Geometry check sheet. Reference: the model listing, model coordinates, mm. A direction names the side the tool comes from. Give positions to 0.01 mm unless a question says otherwise; leave off trailing zeros. Order: outer loops, then holes, each group sorted by start corner. A loop starts at its lowest first (then second) coordinate and runs counter-clockwise, first axis right, second up.
Autodesk Inventor part; units mm, degrees
ref_plane "YZ Plane" through (0, 0, 0) normal (1, 0, 0) x (0, 1, 0)
ref_plane "XZ Plane" through (0, 0, 0) normal (0, 1, 0) x (-1, 0, 0)
ref_plane "XY Plane" through (0, 0, 0) normal (0, 0, 1) x (1, 0, 0)
sketch "Sketch1" plane through (0, 0, 0) normal (0, 1, 0) x (-1, 0, 0)
  line L0 (-12, 184.4696) -> (80, 184.4696)
  line L1 (80, 184.4696) -> (80, -38.9934)
  line L2 (80, -38.9934) -> (-12, -38.9934)
  line L3 (-12, -38.9934) -> (-12, 184.4696)
  point P0 (0, 0)
  dimension "d0" = 92
  dimension "d1" = 223.463
extrude "Extrusion1" add sketch "Sketch1" along normal blind 5
sketch "Sketch2" plane through (0, 5, 0) normal (0, 1, 0) x (1, 0, 0)
  line L0 (-80, -184.4696) -> (12, -184.4696)
  line L1 (12, -184.4696) -> (-13, -184.4696)
  line L2 (-13, -184.4696) -> (-13, -154.4696)
  circle A0 centre (-13, -154.4696) radius 4.75
  line L3 (-13, -154.4696) -> (-13, -114.4696)
  line L4 (-13, -114.4696) -> (-13, -74.4696)
  line L5 (-13, -74.4696) -> (-13, -34.4696)
  circle A1 centre (-13, -114.4696) radius 4.75
  circle A2 centre (-13, -74.4696) radius 4.75
  circle A3 centre (-13, -34.4696) radius 4.75
  line L6 (-13, -34.4696) -> (-13, 5.5304)
  circle A4 centre (-13, 5.5304) radius 4.75
  point P0 (0, 0)
  dimension "d4" = 25
  dimension "d5" = 30
  dimension "d6" = 9.5
  dimension "d7" = 40
  dimension "d8" = 40
  dimension "d9" = 40
  dimension "d10" = 9.5
  dimension "d11" = 9.5
  dimension "d12" = 9.5
  dimension "d34" = 40
  dimension "d35" = 9.5
extrude "Extrusion2" add sketch "Sketch2" along normal blind 5
sketch "Sketch3" plane through (-13, 10, 154.4696) normal (0, 1, 0) x (1, 0, 0)
  circle A0 centre (0, 0) radius 2.5
  circle A1 centre (0, 0) radius 4.75
  line L0 (0, 0) -> (0, 193.463)
  line L1 (25, 193.463) -> (-67, 193.463)
  circle A2 centre (0, 40) radius 2.5
  circle A3 centre (0, 80) radius 2.5
  circle A4 centre (0, 120) radius 2.5
  point P0 (13, 154.4696)
  dimension "d15" = 5
  dimension "d18" = 40
extrude "Extrusion3" cut sketch "Sketch3" against normal blind 3 contours A0 | A4 L0 | L0 A4 | A3 L0 | L0 A3 | A2 L0 | L0 A2
sketch "Sketch4" plane through (0, 5, 0) normal (0, 1, 0) x (1, 0, 0)
  circle A0 centre (-13, -154.4696) radius 2.5
  line L0 (-13, -154.4696) -> (-80, -154.4696)
  line L1 (-80, 38.9934) -> (-80, -184.4696)
  line L2 (-40, -161.9696) -> (-80, -161.9696)
  line L3 (-80, -161.9696) -> (-80, -146.9696)
  line L4 (-80, -146.9696) -> (-40, -146.9696)
  line L5 (-40, -146.9696) -> (-40, -161.9696)
  line L6 (-40, -161.9696) -> (-80, -146.9696) construction
  line L7 (-80, -161.9696) -> (-40, -146.9696) construction
  line L8 (-80, -161.9696) -> (-38.6907, -161.9696)
  line L9 (-38.6907, -161.9696) -> (-38.6907, -171.9696)
  line L10 (-38.6907, -171.9696) -> (-80, -171.9696)
  line L11 (-80, -171.9696) -> (-80, -161.9696)
  line L12 (-80, -146.9696) -> (-38.6907, -146.9696)
  line L13 (-38.6907, -146.9696) -> (-38.6907, -136.9696)
  line L14 (-38.6907, -136.9696) -> (-80, -136.9696)
  line L15 (-80, -136.9696) -> (-80, -146.9696)
  point P0 (0, 0)
  point P1 (-60, -154.4696)
  point P2 (-40.5122, -103.5066)
  point P3 (-80, -136.9696)
  point P4 (-40.5122, -118.5066)
  point P5 (-80, -171.9696)
  point P6 (-40, -146.9696)
  point P7 (-40, -146.9696)
  point P8 (-40, -161.9696)
  dimension "d25" = 15
  dimension "d26" = 40
  dimension "d27" = 10
  dimension "d28" = 10
extrude "Extrusion4" add sketch "Sketch4" along normal blind 5 contours L4 L1 L14 L13 L12 | L8 L9 L10 L1 L2
pattern_linear "Rectangular Pattern1" count 3 spacing 80 along (0, 0, -1) of "Extrusion4"
properties part number "Podstawka"
Item 1: Set-up check for faces 5 (the flat face through (-59, 7, 56.97)), 6 (the flat face through (-13, 7, 34)), 7 (the flat face through (-33, 0, 74)), 8 (the flat face through (-38.691, 7, 167)), 9 (the flat face through (-60, 10, 167)): record each of +Z, -Z, +X, -X, +Y, -Y from which the full face is reachable in a straight line by a thin tool's end or side.
Reported:
face 5: +X, -X, +Y
face 6: +Y
face 7: +Z, -Z, +X, -X, -Y
face 8: +Z, -Z, +X, +Y
face 9: +Z, -Z, +X, -X, +Y
Item 2: Gauge pin test, flat ends, axial feed: pin 1 (1.5 mm diameter, centred on y = 7, z = 86.5, fed in from +X); pin 2 (3 mm diameter, centred on y = 8, z = 21, fed in from +X); pin 3 (4 mm diameter, centred on x = -13, z = 34.47, fed in from +Y); pin 4 (10 mm diameter, centred on x = -30, z = 133, fed in from +Y). Record the tip position at first contact, or that the pin passes through.
Reported:
pin 1: stops at x = -38.69
pin 2: passes through
pin 3: stops at y = 7
pin 4: stops at y = 5
Item 3: Sectioned sample at B-B (x = -64). Enter the section's corners in (y, z), and give its area (3 significant figures).
Reported:
outline: (0, -38.99) - (5, -38.99) - (5, -23.03) - (10, -23.03) - (10, -13.03) - (5, -13.03) - (5, 1.97) - (10, 1.97) - (10, 11.97) - (5, 11.97) - (5, 56.97) - (10, 56.97) - (10, 66.97) - (5, 66.97) - (5, 81.97) - (10, 81.97) - (10, 91.97) - (5, 91.97) - (5, 136.97) - (10, 136.97) - (10, 146.97) - (5, 146.97) - (5, 161.97) - (10, 161.97) - (10, 171.97) - (5, 171.97) - (5, 184.47) - (0, 184.47) - close
area: 1,420 mm2
Item 4: Scan lines: L1, parallel to Z at x = -65.5, y = 7; L2, parallel to X at y = 7.5, z = 74; L3, parallel to X at y = 9, z = 167.5. Record each from-to range of solid material in increasing order.
Reported:
L1: z = -23.03 to -13.03, 1.97 to 11.97, 56.97 to 66.97, 81.97 to 91.97, 136.97 to 146.97, 161.97 to 171.97
L2: x = -17.73 to -15.46, -10.54 to -8.27
L3: x = -80 to -38.69
Item 5: Sectioned sample at C-C (z = 49). Enter the section's corners in (x, y), and give its area (3 significant figures).
Reported:
outline: (-80, 0) - (12, 0) - (12, 5) - (-80, 5) - close
area: 460 mm2
Item 6: Sectioned sample at A-A (y = 8.5). Give the number of separate pieces and of enclosed holes in the cut face, and give its area (3 significant figures).
Reported:
separate pieces: 11
enclosed holes: 4
area: 2,750 mm2
Item 7: Draft check along X on faces 1 (the flat face through (-38.691, 7, 62)), 2 (the flat face through (-35, 2, -38.993)), 3 (the cylindrical face through (-13.54, 8.52, 76.91)), 4 (the cylindrical face through (-14.03, 7.465, -10.167)). Enter one of: released by +X, released by -X, zero draft, split by the parting line, or undercut.
Reported:
face 1: released by +X
face 2: zero draft
face 3: undercut
face 4: split by the parting line
